Check sheet for the modelled part. Datum: model origin and axes. Units: mm. A direction names the side the tool comes from. Give positions to 0.01 mm unless a question says otherwise; leave off trailing zeros. Order: outer loops, then holes, each group sorted by start corner. A loop starts at its lowest first (then second) coordinate and runs counter-clockwise, first axis right, second up.
Item 1: Sectioned sample at A-A on z = 22. Record the boundary of the cut face in (x, y), and give its area (3 significant figures).
Item 2: Gauge pin test, flat ends, axial feed: P1, Ø7.5, axis at x = -2.5, y = -2, coming from the +Z side; P2, Ø10, axis at y = 9, z = 30, coming from the -X side; P3, Ø1, axis at x = 5.5, z = 12, coming from the -Y side; P4, Ø8, axis at x = -3, z = 35, coming from the -Y side. Record the tip position at first contact, or that the pin passes through.
Item 3: Sectioned sample at B-B on z = 9.5. Record the boundary of the cut face in (x, y).
Item 4: Material ranges on line 1 along Y through (x, z) = (0, 3); line 2 along Z through (x, y) = (2.5, 9.5); line 3 along X through (y, z) = (0, 49.5), recorded low to high.
Item 5: Release check for a two-part mould opening along Y. For faces 1 (the flat face through (-3, 8, 49.7)), 2 (the flat face through (0, -6, 48)), 3 (the cylindrical face through (-14.985, 0.66, 23.664)) record: released by +Y, released by -Y, zero draft, split by the parting line, or undercut.
Item 6: Access from +Z, -Z, +X, -X, +Y, -Y to the whole of each face (thin tool, end or side, straight path). Record for faces 4 (the flat face through (3, -7, 49)), 5 (the flat face through (0, 4, 49.4)), 6 (the cylindrical face through (-2.003, -0.631, 5.273)), 7 (the flat face through (3, 0, 0)).
from build123d import *

# Parameters (mm, degrees)
F0_R      = 15
F1_DEPTH  = 50
F2_R      = 2
F3_R      = 10
F4_DEPTH  = 0.3
F6_DEPTH  = 2
F8_D      = 4.2
F8_DEPTH  = 10.4
F8_TIP    = 1.2618073
F9_R      = 8
F10_DEPTH = 0.3


with BuildPart() as f1:
    # F0 (on Top) → F1 (new body)
    with BuildSketch(Plane.XY):
        Circle(F0_R)
    extrude(amount=F1_DEPTH)

    # F2
    f2_edges = [f1.edges().sort_by_distance(p)[0] for p in [
        (-15, 0, 50),
    ]]
    fillet(f2_edges, radius=F2_R)

    # F3 (on face) → F4 (cut)
    with BuildSketch(Plane.XY.offset(50)):
        Circle(F3_R)
    extrude(amount=-F4_DEPTH, mode=Mode.SUBTRACT)

    # F5 (on face) → F6 (cut)
    with BuildSketch(Plane.XY.offset(50)):
        with BuildLine():
            Line((-3, 0), (-3, -9.5393920142))
            ThreePointArc((-3, -9.5393920142), (0, -10), (3, -9.5393920142))
            Line((3, -9.5393920142), (3, 0))
            ThreePointArc((3, 0), (2.1213203436, 2.1213203436), (0, 3))
            ThreePointArc((0, 3), (-2.1213203436, 2.1213203436), (-3, 0))
        make_face()
        with BuildLine():
            Line((-3, -9.5393920142), (-3, -12.6491106407))
            ThreePointArc((-3, -12.6491106407), (0, -13), (3, -12.6491106407))
            Line((3, -12.6491106407), (3, -9.5393920142))
            ThreePointArc((3, -9.5393920142), (0, -10), (-3, -9.5393920142))
        make_face()
        with BuildLine():
            Line((-3, -12.6491106407), (-3, -27))
            Line((-3, -27), (3, -27))
            Line((3, -27), (3, -12.6491106407))
            ThreePointArc((3, -12.6491106407), (0, -13), (-3, -12.6491106407))
        make_face()
    extrude(amount=-F6_DEPTH, mode=Mode.SUBTRACT)

    # F8
    with Locations(Plane(origin=(0, 0, 0), x_dir=(1, 0, 0), z_dir=(0, 0, -1))):
        with Locations((0, 0)):
            Hole(F8_D / 2, depth=F8_DEPTH)
            with Locations((0, 0, -(F8_DEPTH + F8_TIP / 2))):  # 118° drill point
                Cone(0, F8_D / 2, F8_TIP, mode=Mode.SUBTRACT)

    # F9 (on face) → F10 (cut)
    with BuildSketch(Plane.XY.offset(49.7)):
        Circle(F9_R)
    extrude(amount=-F10_DEPTH, mode=Mode.SUBTRACT)


solid = f1.part
Report:
1. outline: circle Ø30 at (0, 0)
1. area: 707 mm2
2. P1: stops at z = 49.4
2. P2: stops at x = -14.46
2. P3: stops at y = -14.14
2. P4: stops at y = -15
3. outline: circle Ø30 at (0, 0); hole circle Ø4.2 at (0, 0)
4. line 1: y = -15 to -2.1, 2.1 to 15
4. line 2: z = 0 to 49.7
4. line 3: x = -14.32 to -8, 8 to 14.32
5. face 1: undercut
5. face 2: zero draft
5. face 3: split by the parting line
6. face 4: +Z, -Y
6. face 5: +Z
6. face 6: -Z
6. face 7: -Z, +X, -X, +Y, -Y
